Here's how the part is built. I have some questions about the finished solid (model axes, mm). Face numbers are marked on the shaded views. A direction names the side the tool comes from. Give positions to 0.01 mm unless a question says otherwise; leave off trailing zeros. Write each loop counter-clockwise with the first axis right and the second up, starting at its lowest first coordinate (ties: lowest second). Pieces come first, ordered by that corner, then holes. Notation, with made-up numbers: M -26,86.5 L 32,86.5 A13 cw 32,97.5 Z; hole C 77.5,-26.75 d11. An arc over 180 degrees is marked long. Use one line per item in the form item = value. Start each with the question number.
from build123d import *

# Parameters (mm, degrees)
CROQUIS1_W              = 82
CROQUIS1_H              = 3.5
SALIENTE_EXTRUIR1_DEPTH = 3.5
CROQUIS2_W              = 15
CROQUIS2_H              = 3.5
CROQUIS2_W_2            = 9
SALIENTE_EXTRUIR2_DEPTH = 22.4
CROQUIS3_W              = 10
CROQUIS3_H              = 3.5
SALIENTE_EXTRUIR3_DEPTH = 36


with BuildPart() as part:
    # Croquis1 → Saliente-Extruir1 (new body)
    with BuildSketch(Plane.XY):
        with Locations((-17.772529993, -26.701946472)):
            Rectangle(CROQUIS1_W, CROQUIS1_H)
    extrude(amount=SALIENTE_EXTRUIR1_DEPTH)

    # Croquis2 → Saliente-Extruir2 (add)
    with BuildSketch(Plane(origin=(0, -24.951946472, 0), x_dir=(1, 0, 0), z_dir=(0, 1, 0))):
        with Locations((15.727470007, -1.75)):
            Rectangle(CROQUIS2_W, CROQUIS2_H)
        with Locations((-54.272529993, -1.75)):
            Rectangle(CROQUIS2_W_2, CROQUIS2_H)
    extrude(amount=SALIENTE_EXTRUIR2_DEPTH)

    # Croquis3 → Saliente-Extruir3 (add)
    with BuildSketch(Plane.XY.offset(3.5)):
        with Locations((-53.772529993, -26.701946472)):
            Rectangle(CROQUIS3_W, CROQUIS3_H)
        with Locations((-17.772529993, -26.701946472)):
            Rectangle(CROQUIS3_W, CROQUIS3_H)
        with Locations((18.227470007, -26.701946472)):
            Rectangle(CROQUIS3_W, CROQUIS3_H)
    extrude(amount=SALIENTE_EXTRUIR3_DEPTH)


solid = part.part
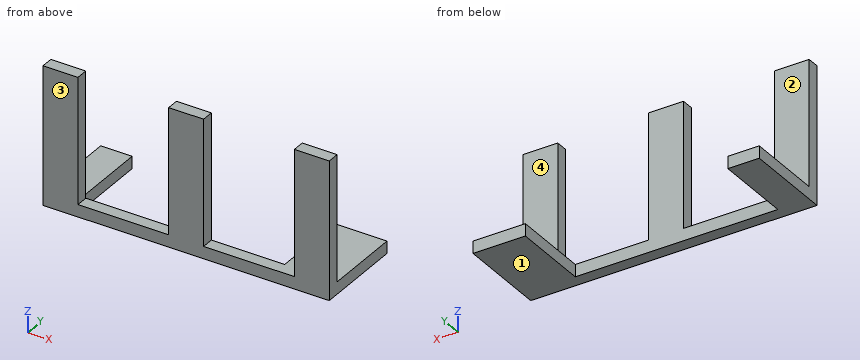
1) On a 3-axis mill with a long thin cutter (end or side, diameter ignored), from which of +Z, -Z, +X, -X, +Y, -Y can I reach the whole of each face in a straight line? I mean the marked faces 3 and 4. Say none if no direction works.
2) Suppose I cut it at D-D, the plane x = -31. List the corners of the cut face in (y, z) for me, and give its area (4 significant figures).
3) Thinking about a two-plate mould opening in X: for the marked faces 1 and 2, which applies, released by +X, released by -X, zero draft, split by the parting line, or undercut?
4) Will these pins go through, and if not, where does the flat tip stop? P1, Ø3, axis at x = 18, z = 22.5, coming from the +Y side; P2, Ø2, axis at x = -23.5, y = -24, coming from the +Z side; P3, Ø10, axis at x = -49, y = -9, coming from the -Z side; P4, Ø10, axis at x = -8, y = -17, coming from the -Z side.
5) Suppose I cut it at A-A, the plane y = -8.5. List the corners of the cut face in (x, z) for me, and give its area (3 significant figures).
6) Please list where these lines run through material, in increasing order: line 1 (X direction, y = -26.75, z = 25); line 2 (X direction, y = -20, z = 2.5); line 3 (Y direction, x = -53.5, z = 15).
7) Suppose I cut it at B-B, the plane z = 12.5. List the corners of the cut face in (x, y) for me.
8) Suppose I cut it at C-C, the plane y = -26. List the corners of the cut face in (x, z) for me.
Checks:
q1.face_3 = +Z, -Z, +X, -X, -Y
q1.face_4 = +Z, +X, -X, +Y
q2.outline = M -28.45,0 L -24.95,0 L -24.95,3.5 L -28.45,3.5 Z
q2.area = 12.25 mm^2
q3.face_1 = zero draft
q3.face_2 = undercut
q4.P1 = -24.95
q4.P2 = 3.5
q4.P3 = 0
q4.P4 = through
q5.outline = M -58.77,0 L -49.77,0 L -49.77,3.5 L -58.77,3.5 Z; M 8.23,0 L 23.23,0 L 23.23,3.5 L 8.23,3.5 Z
q5.area = 84.0 mm^2
q6.line_1 = -58.77 to -48.77, -22.77 to -12.77, 13.23 to 23.23
q6.line_2 = -58.77 to -49.77, 8.23 to 23.23
q6.line_3 = -28.45 to -24.95
q7.outline = M -58.77,-28.45 L -48.77,-28.45 L -48.77,-24.95 L -58.77,-24.95 Z; M -22.77,-28.45 L -12.77,-28.45 L -12.77,-24.95 L -22.77,-24.95 Z; M 13.23,-28.45 L 23.23,-28.45 L 23.23,-24.95 L 13.23,-24.95 Z
q8.outline = M -58.77,0 L 23.23,0 L 23.23,39.5 L 13.23,39.5 L 13.23,3.5 L -12.77,3.5 L -12.77,39.5 L -22.77,39.5 L -22.77,3.5 L -48.77,3.5 L -48.77,39.5 L -58.77,39.5 Z
